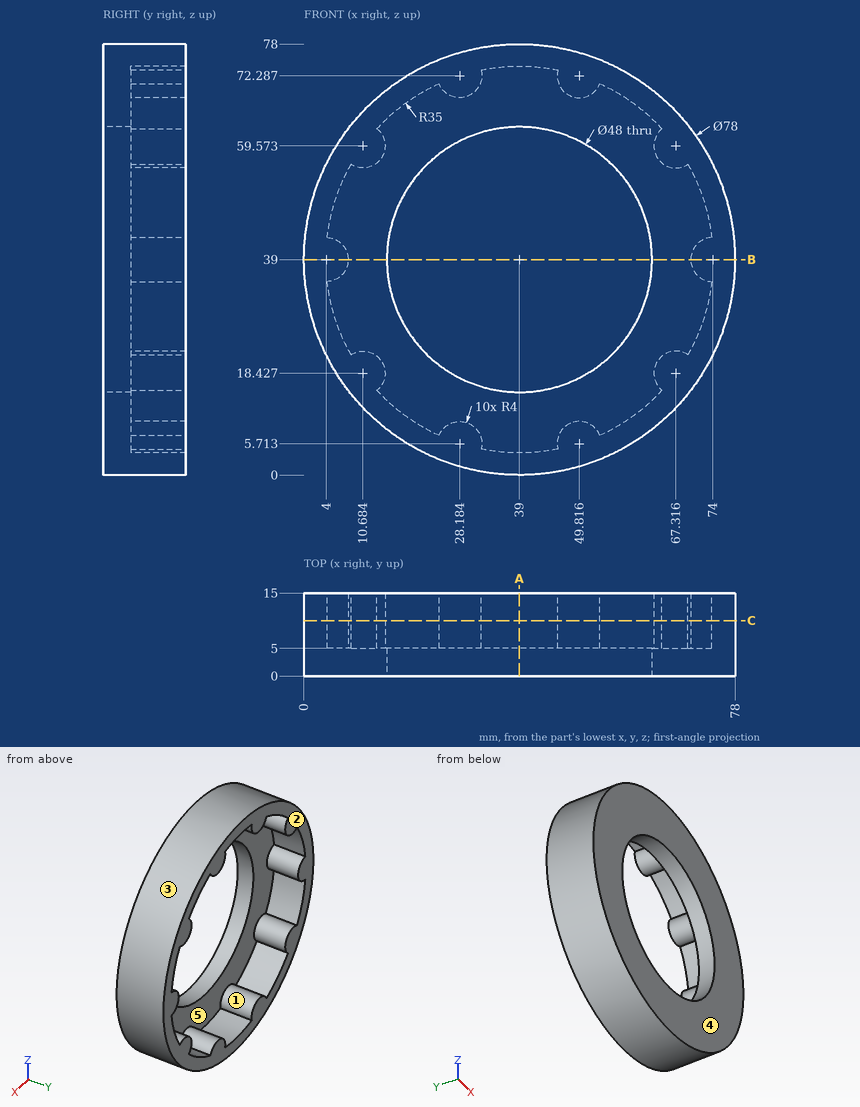
Can you work these out from the drawing? Everything is in mm from the part's minimum corner. A direction names the side the tool comes from. Round coordinates to 2 decimals unless told otherwise and drop trailing zeros. Order: outer loops, then holes, each group sorted by start corner. A loop starts at its lowest first (then second) coordinate and runs counter-clockwise, first axis right, second up. Notation, with made-up numbers: M 89,-6 L 106,-6 A23 ccw 106,2 Z; hole C 58,-21 d9. An arc over 180 degrees is marked long. One line per question, with ' | ' between items.
1) I want a section at B-B, the plane z = 39. Write out the boundary of the cut face in (x, y), then the cut area to 3 significant figures.
Working result:
outline: M 0,0 L 15,0 L 15,5 L 8,5 L 8,15 L 0,15 Z; M 63,0 L 78,0 L 78,15 L 70,15 L 70,5 L 63,5 Z | area: 310 mm²
2) For pin 1 Ø1.5 at (y, z) = (12.5, 12) entering from +X (1 decimal); pin 2 Ø6 at (x, y) = (21, 2) entering from -Z; pin 3 Ø4 at (y, z) = (3, 9.5) entering from -X (1 decimal), each with a flat end and sliding along its axis, tell me the tip position at first contact or that it passes through.
Working result:
pin 1: x = 67.8 | pin 2: z = 3 | pin 3: x = 11.3
3) If we mould it in two halves opening along X, with no side actions, what happens to the marked faces 1, 2 and 3? For each: +X half, -X half, draft (parallel to the pull), parting line (faces both ways), or undercut.
Working result:
face 1: undercut | face 2: draft | face 3: parting line
4) For the marked faces 4 and 5, which set-ups out of +Z, -Z, +X, -X, +Y, -Y let a thin tool reach every point of the face, with its end or its side?
Working result:
face 4: +Z, -Z, +X, -X, -Y | face 5: +Y
5) I want a section at C-C, the plane y = 10. Write out the boundary of the cut face in (x, z) (1 decimal).
Working result:
outline: C 39,39 d78; hole M 4.2,35 A35 ccw 8.5,21.8 A4 cw 13.2,15.3 A35 ccw 24.5,7.2 A4 cw 32.1,4.7 A35 ccw 45.9,4.7 A4 cw 53.5,7.2 A35 ccw 64.8,15.3 A4 cw 69.5,21.8 A35 ccw 73.8,35 A4 cw 73.8,43 A35 ccw 69.5,56.2 A4 cw 64.8,62.7 A35 ccw 53.5,70.8 A4 cw 45.9,73.3 A35 ccw 32.1,73.3 A4 cw 24.5,70.8 A35 ccw 13.2,62.7 A4 cw 8.5,56.2 A35 ccw 4.2,43 A4 cw Z
6) I want a section at A-A, the plane x = 39. Write out the boundary of the cut face in (y, z).
Working result:
outline: M 0,0 L 15,0 L 15,4 L 5,4 L 5,15 L 0,15 Z; M 0,63 L 5,63 L 5,74 L 15,74 L 15,78 L 0,78 Z
7) I need wall thicknesses on line 1 along Z through (x, y) = (39, 4); line 2 along Y through (x, z) = (18.5, 19.5); line 3 along X through (y, z) = (8.5, 55) (1 decimal). Which ranges of each line are inside material? Lowest first, please.
Working result:
line 1: 0 to 15, 63 to 78 | line 2: 0 to 5 | line 3: 3.4 to 7.9, 70.1 to 74.6
